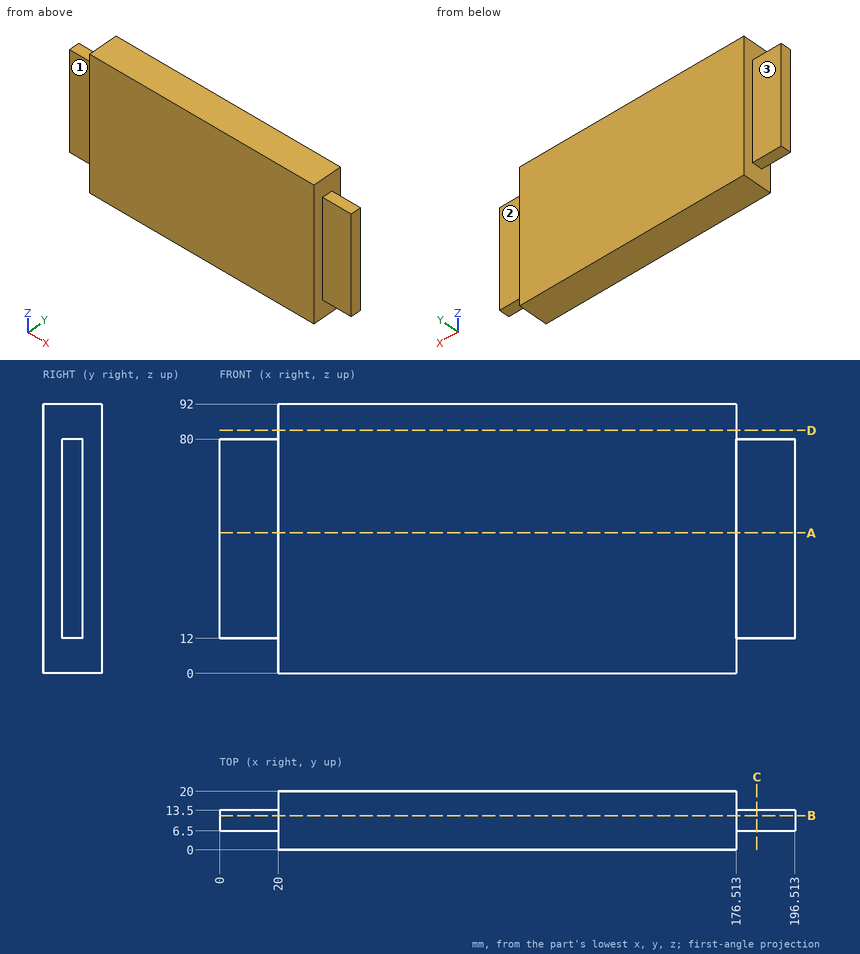
Geometry check sheet. Reference: drawing and pictorial views, mm from the part's lowest x, y, z. A direction names the side the tool comes from. Round coordinates to 2 decimals unless told otherwise and drop trailing zeros. Order: outer loops, then holes, each group sorted by start corner. A loop starts at its lowest first (then second) coordinate and runs counter-clockwise, first axis right, second up. Notation, with made-up numbers: (-36.75, 40) -> (-8.75, 40) arc R13 ccw to (-8.75, 45) -> close; hole circle Ø1 at (74.25, 3.5). An arc over 180 degrees is marked (long way). One line per item, written item: value. Start each with the question number.
Q1. Set-up check for the marked faces 1, 2 and 3: record each of +Z, -Z, +X, -X, +Y, -Y from which the full face is reachable in a straight line by a thin tool's end or side.
Q2. Cross-section at D-D (z = 83). Record the boundary of the cut face in (x, y), and give its area (3 significant figures).
Q3. Thickness scan on line 1 (X direction, y = 4.75, z = 30); line 2 (Y direction, x = 180, z = 63); line 3 (Z direction, x = 11, y = 12.75). Record the ranges inside material, lowest first.
Q4. Cross-section at C-C (x = 183.5). Record the boundary of the cut face in (y, z).
Q5. Gauge pin test, flat ends, axial feed: pin 1 Ø12 at (y, z) = (13.5, 12.5) entering from -X; pin 2 Ø2 at (x, y) = (189.5, 8.5) entering from +Z; pin 3 Ø2 at (y, z) = (18, 56) entering from -X; pin 4 Ø7.5 at (x, y) = (6, 11.5) entering from -Z. Record the tip position at first contact, or that the pin passes through.
Q6. Cross-section at A-A (z = 48). Record the boundary of the cut face in (x, y).
Q7. Cross-section at B-B (y = 11.75). Record the boundary of the cut face in (x, z).
Completed:
1. face 1: +Z, -Z, -X, -Y
1. face 2: +Z, -Z, +X, +Y
1. face 3: +Z, -Z, -X, +Y
2. outline: (20, 0) -> (176.51, 0) -> (176.51, 20) -> (20, 20) -> close
2. area: 3,130 mm²
3. line 1: x = 20 to 176.51
3. line 2: y = 6.5 to 13.5
3. line 3: z = 12 to 80
4. outline: (6.5, 12) -> (13.5, 12) -> (13.5, 80) -> (6.5, 80) -> close
5. pin 1: stops at x = 0
5. pin 2: stops at z = 80
5. pin 3: stops at x = 20
5. pin 4: stops at z = 12
6. outline: (0, 6.5) -> (20, 6.5) -> (20, 0) -> (176.51, 0) -> (176.51, 6.5) -> (196.51, 6.5) -> (196.51, 13.5) -> (176.51, 13.5) -> (176.51, 20) -> (20, 20) -> (20, 13.5) -> (0, 13.5) -> close
7. outline: (0, 12) -> (20, 12) -> (20, 0) -> (176.51, 0) -> (176.51, 12) -> (196.51, 12) -> (196.51, 80) -> (176.51, 80) -> (176.51, 92) -> (20, 92) -> (20, 80) -> (0, 80) -> close
